Part model, mm, in its own coordinate system. Round coordinates to 2 decimals unless told otherwise and drop trailing zeros. Write each loop counter-clockwise with the first axis right and the second up, starting at its lowest first coordinate (ties: lowest second). Pieces come first, ordered by that corner, then holes. Notation, with made-up numbers: M 21,-11 L 29,-11 A11 cw 29,4 Z; hole C 85.5,19.5 d9. An arc over 180 degrees is marked long. Use a Markdown table: item, result. Add a question column.
1) Slice it at B-B on z = -11. Give the number of separate pieces and of enclosed holes in the cut face, plus the area to 3 significant figures.
2) Two-plate mould, pull along Z, no slides. Class faces 1 (the face through (-19.524, 9.888, -4.336)), 2 (the face through (37.945, 9.888, -42.793)), 3 (the face through (37, 0, -15)): released by +Z, released by -Z, zero draft, split by the parting line, or undercut.
3) Wall check: probe 1 along X at (y, z) = (13.75, -11); probe 2 along X at (y, z) = (6.5, -6); probe 3 along X at (y, z) = (3.25, -23.5). Give the ranges that are in metal, low to high.
4) Drop flat-ended pins along their axis: P1, Ø1.5, axis at y = 3, z = -34.5, coming from the -X side; P2, Ø3, axis at x = -3.5, z = -18.5, coming from the +Y side; P3, Ø1.5, axis at x = 52, y = 15.5, coming from the -Z side. Give the stop position or say it passes through.
5) Slice it at A-A on y = 12. Write the cut outline in (x, z) (3 decimals), plus the area to 3 significant figures.
```python
from build123d import *

# Parameters (mm, degrees)
CROQUIS2_R              = 20
CROQUIS2_R_2            = 12.5
SALIENTE_EXTRUIR1_DEPTH = 20
CHAFL_N1_SIZE           = 2


with BuildPart() as part:
    # Croquis2 → Saliente-Extruir1 (new body)
    with BuildSketch(Plane(origin=(0, 0, 0), x_dir=(1, 0, 0), z_dir=(0, 1, 0))):
        with BuildLine():
            ThreePointArc((-15.269779386, 25.823126021), (-23.871178313, -18.170493828), (20.824407657, -21.59500048))
            ThreePointArc((20.824407657, -21.59500048), (48.893723191, -5.058826483), (81.407845118, -3.018385264))
            ThreePointArc((81.407845118, -3.018385264), (104.144121582, 11.476569523), (91.783061927, 35.440003874))
            ThreePointArc((91.783061927, 35.440003874), (37.170213372, 42.72542693), (-15.269779386, 25.823126021))
        make_face()
        with Locations(Location((0, 0, 0), (0, 0, 270))):
            Circle(CROQUIS2_R, mode=Mode.SUBTRACT)
        with Locations(Location((84.83446024, 16.68588607, 0), (0, 0, 270))):
            Circle(CROQUIS2_R_2, mode=Mode.SUBTRACT)
    extrude(amount=SALIENTE_EXTRUIR1_DEPTH)

    # Chaflán1
    chafl_n1_edges = [part.edges().sort_by_distance(p)[0] for p in [
        (0, 0, -20),
        (0, 20, -20),
        (37.170213372, 20, -42.72542693),
        (84.83446024, 0, -29.18588607),
        (84.83446024, 20, -29.18588607),
        (-23.871178313, 20, 18.170493828),
        (48.893723191, 20, 5.058826483),
        (-23.871178313, 0, 18.170493828),
        (37.170213372, 0, -42.72542693),
        (104.144121582, 0, -11.476569523),
        (48.893723191, 0, 5.058826483),
        (104.144121582, 20, -11.476569523),
    ]]
    chamfer(chafl_n1_edges, length=CHAFL_N1_SIZE)


solid = part.part
```
Entries:
| question | item | result |
|---|---|---|
| 1 | separate pieces | 3 |
| 1 | enclosed holes | 0 |
| 1 | area | 1,500 mm^2 |
| 2 | face 1 | undercut |
| 2 | face 2 | released by -Z |
| 2 | face 3 | zero draft |
| 3 | probe 1 | x = -27.91 to -16.7, 16.7 to 73.7, 95.97 to 104.01 |
| 3 | probe 2 | x = -29.39 to -19.08, 19.08 to 78.35, 91.32 to 101.74 |
| 3 | probe 3 | x = -18.65 to 74.36, 95.31 to 103.64 |
| 4 | P1 | stops at x = 0.61 |
| 4 | P2 | stops at y = 18.33 |
| 4 | P3 | stops at z = -43.19 |
| 5 | outline | M -15.27,-25.823 A125 ccw 91.783,-35.44 A20 ccw 81.408,3.018 A70 cw 20.824,21.595 A30 ccw long Z; hole C 0,0 d40; hole C 84.834,-16.686 d25 |
| 5 | area | 4,770 mm^2 |
